Could you check a few things on this model? Use its own coordinates, in mm. Face numbers are marked on the shaded views. A direction names the side the tool comes from. Round coordinates to 2 decimals unless told otherwise and drop trailing zeros. Loops run counter-clockwise (first coordinate to the right, second up) from the corner with the lowest first, then second, coordinate; pieces in that order, holes last. Notation, with made-up numbers: (48, 81) -> (58, 81) arc R12 cw to (58, 89) -> close; hole circle Ø11 at (-15, 72). An arc over 180 degrees is marked (long way). One line per item, written item: value.
from build123d import *

# Parameters (mm, degrees)
SKETCH1_R           = 3
BOSS_EXTRUDE1_DEPTH = 5
SKETCH2_R           = 2.5
CUT_EXTRUDE1_DEPTH  = 4
SKETCH3_R           = 4
BOSS_EXTRUDE3_DEPTH = 1
FILLET2_R           = 1
FILLET3_R           = 4


# Some blends are built 0.0001 mm under size
with BuildPart() as part:
    # Sketch1 → Boss-Extrude1 (new body)
    with BuildSketch(Plane(origin=(0, 0, 0), x_dir=(1, 0, 0), z_dir=(0, 1, 0))):
        with Locations(Location((0, 0, 0), (0, 0, 270))):
            Circle(SKETCH1_R)
    extrude(amount=BOSS_EXTRUDE1_DEPTH)

    # Sketch2 → Cut-Extrude1 (cut)
    with BuildSketch(Plane(origin=(0, 5, 0), x_dir=(1, 0, 0), z_dir=(0, 1, 0))):
        with Locations(Location((0, 0, 0), (0, 0, 270))):
            Circle(SKETCH2_R)
    extrude(amount=-CUT_EXTRUDE1_DEPTH, mode=Mode.SUBTRACT)

    # Sketch3 → Boss-Extrude3 (add)
    with BuildSketch(Plane.XZ):
        with Locations(Location((0, 0, 0), (0, 0, 270))):
            Circle(SKETCH3_R)
    extrude(amount=BOSS_EXTRUDE3_DEPTH)

    # Fillet2
    fillet2_edges = [part.edges().sort_by_distance(p)[0] for p in [
        (0, 0, -3),
    ]]
    fillet(fillet2_edges, radius=FILLET2_R - 0.0001)  # a hair under: the kernel refuses the full size

    # Fillet3
    # the kernel refuses this fillet: 4 mm, written as the material it takes off along each edge
    with BuildSketch(Plane(origin=(0, -1, 0), x_dir=(0, 0, -1), z_dir=(-1, 0, 0))) as fillet3_piece_1:
        with BuildLine():
            CenterArc((1.354248689, -4), FILLET3_R, 48.590377891, 41.409622109)
            Line((1.354248689, 0), (1.354248689, 0.08))
            Line((1.354248689, 0.08), (4, 0.08))
            Line((4, 0.08), (4.08, 0))
            ThreePointArc((4.08, 0), (4.08, -0.5), (4.052915026, -0.94))
            Line((4.052915026, -0.94), (4, -1))
        make_face()
    revolve(axis=Axis((0, -1, 0), (0, -1, 0)), mode=Mode.SUBTRACT)


solid = part.part
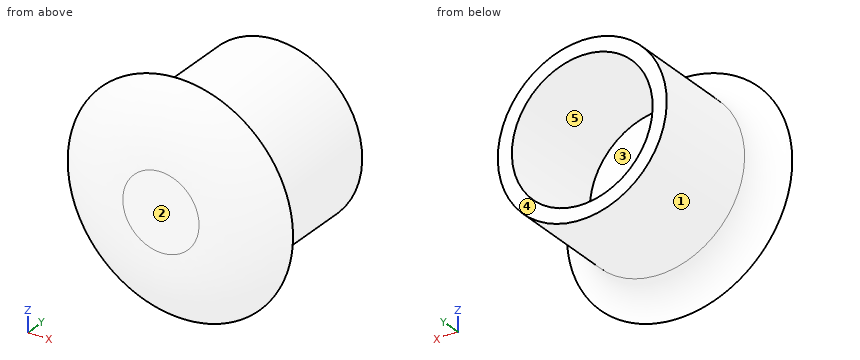
(1) I'm going to push flat-ended pins straight in: pin 1 Ø2 at (x, z) = (0, -2.5) entering from -Y; pin 2 Ø3 at (x, z) = (0, 0) entering from +Y. Where does each tip first touch, or does it pass through?
Recorded:
pin 1: y = -1
pin 2: y = 1
(2) If I drill on L1, parallel to X at y = 2.4, z = 0; L2, parallel to Z at x = -1.5, y = 3; L3, parallel to X at y = 1.25, z = -1.25, over which ranges is the centre line in solid material (lowest first)?
Recorded:
L1: -3 to -2.5, 2.5 to 3
L2: -2.6 to -2, 2 to 2.6
L3: -2.73 to -2.17, 2.17 to 2.73
(3) If we section it at A-A, the plane y = 3: Please give me the cut outline in (x, z), then the cut area to 3 significant figures.
Recorded:
outline: circle Ø6 at (0, 0); hole circle Ø5 at (0, 0)
area: 8.64 mm²
(4) Thinking about a two-plate mould opening in X: for the marked faces 1, 2 and 3, which applies, released by +X, released by -X, zero draft, split by the parting line, or undercut?
Recorded:
face 1: split by the parting line
face 2: zero draft
face 3: undercut
(5) For the marked faces 4 and 5, which set-ups out of +Z, -Z, +X, -X, +Y, -Y let a thin tool reach every point of the face, with its end or its side?
Recorded:
face 4: +Z, -Z, +X, -X, +Y
face 5: +Y
